Autodesk Inventor part; units mm, degrees
ref_plane "Start plane" through (0, 0, 0) normal (0, 0, 1) x (1, 0, 0)
ref_plane "End plane" through (0, 0, 1658) normal (0, 0, 1) x (1, 0, 0)
ref_plane "YZ Plane" through (0, 0, 0) normal (1, 0, 0) x (0, 1, 0)
ref_plane "Start plane" through (0, 0, 0) normal (0, 0, 1) x (1, 0, 0)
ref_plane "End plane" through (0, 0, 1658) normal (0, 0, 1) x (1, 0, 0)
sketch "Sketch" plane through (0, 0, 0) normal (0, 0, 1) x (1, 0, 0)
  line L0 (-9.2, 25) -> (9.2, 25)
  line L1 (15, 19.2) -> (15, -19.2)
  line L2 (9.2, -25) -> (-9.2, -25)
  line L3 (-15, -19.2) -> (-15, 19.2)
  arc A0 (-9.2, 25) -> (-15, 19.2) centre (-9.2, 19.2) ccw
  arc A1 (15, 19.2) -> (9.2, 25) centre (9.2, 19.2) ccw
  arc A2 (9.2, -25) -> (15, -19.2) centre (9.2, -19.2) ccw
  arc A3 (-15, -19.2) -> (-9.2, -25) centre (-9.2, -19.2) ccw
  line L4 (-22.6817, 0) -> (22.6817, 0) construction
  line L5 (0, -36.6817) -> (0, 36.6817) construction
  arc A4 (-9.2, 22.1) -> (-12.1, 19.2) centre (-9.2, 19.2) ccw
  line L6 (-9.2, 22.1) -> (9.2, 22.1)
  arc A5 (12.1, 19.2) -> (9.2, 22.1) centre (9.2, 19.2) ccw
  line L7 (12.1, 19.2) -> (12.1, -19.2)
  arc A6 (9.2, -22.1) -> (12.1, -19.2) centre (9.2, -19.2) ccw
  line L8 (9.2, -22.1) -> (-9.2, -22.1)
  arc A7 (-12.1, -19.2) -> (-9.2, -22.1) centre (-9.2, -19.2) ccw
  line L9 (-12.1, -19.2) -> (-12.1, 19.2)
  point P0 (-15, 25)
  point P1 (15, -25)
  point P2 (15, 25)
  dimension "b" = 30
  dimension "ParH" = 50
  dimension "msp_r" = 5.8
  dimension "d8" = 15
  dimension "d9" = 25
  dimension "d10" = 2.9
extrude "Body" add sketch "Sketch" along normal up to surface (1658 mm away) from surface at 0
sketch "Sketch2" plane through (0, 0, 0) normal (0, 0, 1) x (1, 0, 0)
  line L0 (0, 0) -> (10, 0)
ref_plane "Work Plane3" through (0, 0, 0) normal (0, -1, 0) x (1, 0, 0)
sketch "Sketch3" plane through (0, 0, 0) normal (0, -1, 0) x (1, 0, 0)
  line L0 (-2, 0) -> (12, 0)
  line L1 (-2, 1658) -> (12, 1658)
  dimension "d14" = 1658
equation "\"msp_r\" = 2 * ParT"
equation "\"d8\" = 0.5 * b"
equation "\"d9\" = 0.5 * ParH"
equation "\"d10\" = ParT"
equation "\"G_OFFSET_START\" = 0"
equation "\"G_OFFSET_END\" = 0"
equation "\"d12\" = G_OFFSET_END + B_L"
equation "\"G_L\" = d14"
equation "\"B_L\" = 1658"
properties part number "DIN 59 410 - 50x30x2.9-1658" material "Steel, Mild"
Can you work these out from the model? Positions are in its coordinate system, mm. A direction names the side the tool comes from. Give positions to 0.01 mm unless a question says otherwise; leave off trailing zeros. Loops run counter-clockwise (first coordinate to the right, second up) from the corner with the lowest first, then second, coordinate; pieces in that order, holes last. Notation, with made-up numbers: M -18,19.25 L -4,19.25 A22 cw -4,26.25 Z; hole C 18.25,86 d5. An arc over 180 degrees is marked long. Answer in a Markdown table with one row per item.
1. If I drill on line 1 along X through (y, z) = (2.5, 219.5); line 2 along Y through (x, z) = (7, 690); line 3 along X through (y, z) = (21, 222), over which ranges is the centre line in solid material (lowest first)?
Taken from the geometry:
| item | result |
|---|---|
| line 1 | x = -15 to -12.1, 12.1 to 15 |
| line 2 | y = -25 to -22.1, 22.1 to 25 |
| line 3 | x = -14.71 to -11.47, 11.47 to 14.71 |
2. Suppose I cut it at C-C on z = 811. Write out the boundary of the cut face in (x, y).
Taken from the geometry:
| item | result |
|---|---|
| outline | M -15,-19.2 A5.8 ccw -9.2,-25 L 9.2,-25 A5.8 ccw 15,-19.2 L 15,19.2 A5.8 ccw 9.2,25 L -9.2,25 A5.8 ccw -15,19.2 Z; hole M -12.1,-19.2 A2.9 ccw -9.2,-22.1 L 9.2,-22.1 A2.9 ccw 12.1,-19.2 L 12.1,19.2 A2.9 ccw 9.2,22.1 L -9.2,22.1 A2.9 ccw -12.1,19.2 Z |
3. Suppose I cut it at A-A on y = -3. Write out the boundary of the cut face in (x, z).
Taken from the geometry:
| item | result |
|---|---|
| outline | M -15,0 L -12.1,0 L -12.1,1658 L -15,1658 Z; M 12.1,0 L 15,0 L 15,1658 L 12.1,1658 Z |
4. Thinking about a two-plate mould opening in X: for faces 3 (the flat face through (-12.1, 0, 817)), 4 (the flat face through (-15, 0, 817)), 5 (the flat face through (-12.3, 2, 1658)), which applies, released by +X, released by -X, zero draft, split by the parting line, or undercut?
Taken from the geometry:
| item | result |
|---|---|
| face 3 | undercut |
| face 4 | released by -X |
| face 5 | zero draft |
5. Which directions (+Z, -Z, +X, -X, +Y, -Y) give clear straight access to the entire face, cutting with the end or side of a thin tool? Please do faces 1 (the flat face through (12.1, 0, 817)), 2 (the flat face through (-12.3, 2, 0)).
Taken from the geometry:
| item | result |
|---|---|
| face 1 | +Z, -Z |
| face 2 | -Z, +X, -X, +Y, -Y |
6. Suppose I cut it at B-B on x = 4.5. Write out the boundary of the cut face in (y, z).
Taken from the geometry:
| item | result |
|---|---|
| outline | M -25,0 L -22.1,0 L -22.1,1658 L -25,1658 Z; M 22.1,0 L 25,0 L 25,1658 L 22.1,1658 Z |
7. For pin 1 Ø4 at (x, z) = (-11, 695.5) entering from -Y; pin 2 Ø2 at (x, y) = (-9.5, -15) entering from +Z; pin 3 Ø1 at (x, z) = (-10.5, 1431) entering from -Y, each with a flat end and sliding along its axis, tell me the tip position at first contact or that it passes through.
Taken from the geometry:
| item | result |
|---|---|
| pin 1 | stops at y = -25 |
| pin 2 | passes through |
| pin 3 | stops at y = -24.94 |
